Part model, mm, in its own coordinate system. A direction names the side the tool comes from. Round coordinates to 2 decimals unless told otherwise and drop trailing zeros. Write each loop counter-clockwise with the first axis right and the second up, starting at its lowest first coordinate (ties: lowest second). Pieces come first, ordered by that corner, then holes. Notation, with made-up numbers: (66.25, -32) -> (108.25, -32) arc R33 ccw to (108.25, -2) -> close; hole circle Ø2 at (42.25, 76). An arc over 180 degrees is marked (long way). Return JSON: item names as keys, results as strings. Group by question number.
(1) Drill centre lines: L1, parallel to X at y = 2.4, z = -28; L2, parallel to Z at x = -62.5, y = 0.85; L3, parallel to Z at x = -54.5, y = 2.1. Where is each one in solid material? Low to high. Write a range as from..to.
(2) Drop flat-ended pins along their axis: pin 1 Ø8 at (x, z) = (-31.5, -48) entering from +Y; pin 2 Ø6 at (x, z) = (-64, -63) entering from +Y; pin 3 Ø5 at (x, z) = (-4.83, -64.17) entering from +Y. Give the stop position or say it passes through.
(3) Tool access for faces 4 (the cylindrical face through (-7.073, 5.014, -3.107)), 5 (the flat face through (-19, 0, -26)): list every direction of +Z, -Z, +X, -X, +Y, -Y with a clear straight run to the whole face (end or side of a thin tool).
(4) Saw through at B-B (x = -19). List the corners of the cut face in (y, z), plus the area to 3 significant figures.
(5) Mould opens along Z. For faces 1 (the cylindrical face through (-65.65, 2.03, -65.52)), 2 (the cylindrical face through (-68.43, 1.97, -68.4)), 3 (the flat face through (-69, 2, -34)) say: +Z half, -Z half, draft (parallel to the pull), parting line (faces both ways), or undercut.
(6) Saw through at A-A (z = -29). List the corners of the cut face in (x, y), plus the area to 3 significant figures.
Autodesk Inventor part; units mm, degrees
ref_plane "YZ Plane" through (0, 0, 0) normal (1, 0, 0) x (0, 1, 0)
ref_plane "XZ Plane" through (0, 0, 0) normal (0, 1, 0) x (-1, 0, 0)
ref_plane "XY Plane" through (0, 0, 0) normal (0, 0, 1) x (1, 0, 0)
sketch "Sketch1" plane through (0, 0, 0) normal (0, 1, 0) x (-1, 0, 0)
  line L0 (0, 0) -> (69, 0)
  line L1 (69, 0) -> (69, -69)
  line L2 (69, -69) -> (0, -69)
  line L3 (0, -69) -> (0, 0)
  dimension "d0" = 69
  dimension "d1" = 69
extrude "Extrusion1" add sketch "Sketch1" along normal blind 6
sketch "Sketch2" plane through (0, 6, 0) normal (0, 1, 0) x (1, 0, 0)
  line L0 (0, 0) -> (0, 69) construction
  line L1 (0, 69) -> (-69, 69) construction
  line L2 (0, 0) -> (-69, 69) construction
  line L3 (-69, 69) -> (-69, 0) construction
  line L4 (-69.6585, 0.6585) -> (-0.6585, 69.6585) construction
  circle A0 centre (-37.9036, 37.4036) radius 20
  line L5 (-61.9507, 69) -> (-61.9507, 54) construction
  line L6 (-37.9036, 17.4036) -> (-58.9036, 17.4036) construction
  line L7 (-58.9036, 17.4036) -> (-17.4036, 17.4036) construction
  line L8 (-58.4036, 17.4036) -> (-58.4036, 58.5866) construction
  line L9 (-58.4036, 58.5866) -> (-17.4036, 58.5866) construction
  line L10 (-17.4036, 58.5866) -> (-17.4036, 17.4036) construction
  line L11 (-69, 69) -> (-69, 0) construction
  line L12 (-69, 54) -> (-54, 54) construction
  line L13 (-69, 69) -> (-37.9036, 37.9036)
  dimension "d4" = 40
  dimension "d55" = 15
  dimension "d65" = 43.977
extrude "Extrusion2" cut sketch "Sketch2" against normal blind 6
fillet "Fillet1" radius 2 1 edges at (-34.5, 6, 0)
fillet "Fillet2" radius 2 3 edges at (0, 6, -35.5) (0, 5.4142, -0.5858) (0, 2, 0)
fillet "Fillet3" radius 2 3 edges at (-0.5858, 5.4142, -69) (0, 2, -69) (-35.5, 6, -69)
fillet "Fillet4" radius 2 5 edges at (-69, 5.4142, -0.5858) (-69, 2, 0) (-69, 5.4142, -68.4142) (-69, 2, -69) (-69, 6, -34.5)
sketch "Sketch3" plane through (0, 6, 0) normal (0, 1, 0) x (1, 0, 0)
  line L0 (-67, 69) -> (-67, 67) construction
  line L1 (-2, 2) -> (-67, 2) construction
  line L2 (-67, 67) -> (-2, 67) construction
  line L3 (-67, 2) -> (-67, 67) construction
  circle A0 centre (-22, 53.808) radius 1.25
  line L4 (-69, 67) -> (-69, 2) construction
  circle A1 centre (-37.9036, 37.4036) radius 20 construction
  line L5 (-17.9036, 37.4036) -> (-17.9036, 58.4036) construction
  line L6 (-22, 53.808) -> (-54, 53.808) construction
  line L7 (-22, 21.808) -> (-54, 21.808) construction
  line L8 (-54, 21.808) -> (-54, 53.808) construction
  line L9 (-22, 53.808) -> (-22, 21.808) construction
  line L10 (-22, 53.808) -> (-54, 21.808) construction
  line L11 (-69, 59.0495) -> (-54, 59.0495) construction
  line L12 (-54, 69) -> (-54, 53.808) construction
  point P0 (0, 0)
  dimension "d14" = 2.5
  dimension "d63" = 32
  dimension "d64" = 15
extrude "Extrusion3" cut sketch "Sketch3" against normal blind 10
pattern_circular "Circular Pattern1" count 4 over 360 about axis through (-37.9036, 6, -37.4036) along (0, -1, 0) of "Extrusion3"
sketch "Sketch6" plane through (0, 6, 0) normal (0, 1, 0) x (1, 0, 0)
  line L0 (-2, 67) -> (-2, 2)
  arc A0 (-2, 0) -> (0, 2) centre (-2, 2) ccw
  line L1 (0, 2) -> (-2, 2)
  line L2 (0, 0) -> (-2, 2)
  line L3 (-0.5858, 0.5858) -> (-4.8284, 4.8284) construction
  circle A1 centre (-4.8284, 4.8284) radius 2
  dimension "d52" = 6
  dimension "d53" = 4
extrude "Extrusion5" cut sketch "Sketch6" against normal blind 18.75 contours A1
pattern_linear "Rectangular Pattern1" count 2 spacing 59.343 along (0, 0, -1) count 2 spacing 59.343 along (-1, 0, 0) of "Extrusion5"
sketch "Sketch8" plane through (0, 6, 0) normal (0, 1, 0) x (1, 0, 0)
  line L0 (-2, 2) -> (-67, 2)
  circle A0 centre (-4.8284, 4.8284) radius 2 construction
  line L1 (-4.8284, 4.8284) -> (-2, 2) construction
  circle A1 centre (-4.8284, 4.8284) radius 2.8284 construction
  circle A2 centre (-4.8284, 4.8284) radius 2.8284
  circle A3 centre (-4.8284, 4.8284) radius 2
  point P0 (0, 0)
  point P1 (-4.1213, 4.1213)
extrude "Extrusion6" cut sketch "Sketch8" against normal blind 2 contours A2 | A3
pattern_linear "Rectangular Pattern2" count 2 spacing 59.343 along (-1, 0, 0) count 2 spacing 59.343 along (0, 0, -1) of "Extrusion6"
sketch "Sketch9" plane through (0, 6, 0) normal (0, 1, 0) x (1, 0, 0)
  circle A0 centre (-37.9036, 37.4036) radius 20
  circle A1 centre (-37.9036, 37.4036) radius 26.5
  point P0 (0, 0)
  dimension "d59" = 53
extrude "Extrusion7" cut sketch "Sketch9" against normal blind 2
equation "\"d0\" = d1"
properties part number "joystickBOXtop"
Computed values:
{
 "1": {"L1": "-69..-55.56, -20.25..0", "L2": "-69..-65.27, -63.07..-5.93, -3.73..0", "L3": "-69..-54.54, -52.07..-48.56, -26.24..-22.04, -19.96..0"},
 "2": {"pin 1": "through", "pin 2": "y = 6", "pin 3": "y = 4"},
 "3": {"face 4": "+Y", "face 5": "+Z, -Z, +X, -X, -Y"},
 "4": {"outline": "(0, -69) -> (4, -69) arc R2 ccw to (6, -67) -> (6, -55.98) -> (4, -55.98) -> (4, -43.93) -> (0, -43.93) -> close; (0, -30.87) -> (4, -30.87) -> (4, -18.83) -> (6, -18.83) -> (6, -2) arc R2 ccw to (4, 0) -> (0, 0) -> close", "area": "286 mm2"},
 "5": {"face 1": "undercut", "face 2": "-Z half", "face 3": "draft"},
 "6": {"outline": "(-69, 0) -> (-56.05, 0) -> (-56.05, 4) -> (-63.04, 4) -> (-63.04, 6) -> (-67, 6) arc R2 ccw to (-69, 4) -> close; (-19.75, 0) -> (0, 0) -> (0, 4) arc R2 ccw to (-2, 6) -> (-12.77, 6) -> (-12.77, 4) -> (-19.75, 4) -> close", "area": "167 mm2"}
}
